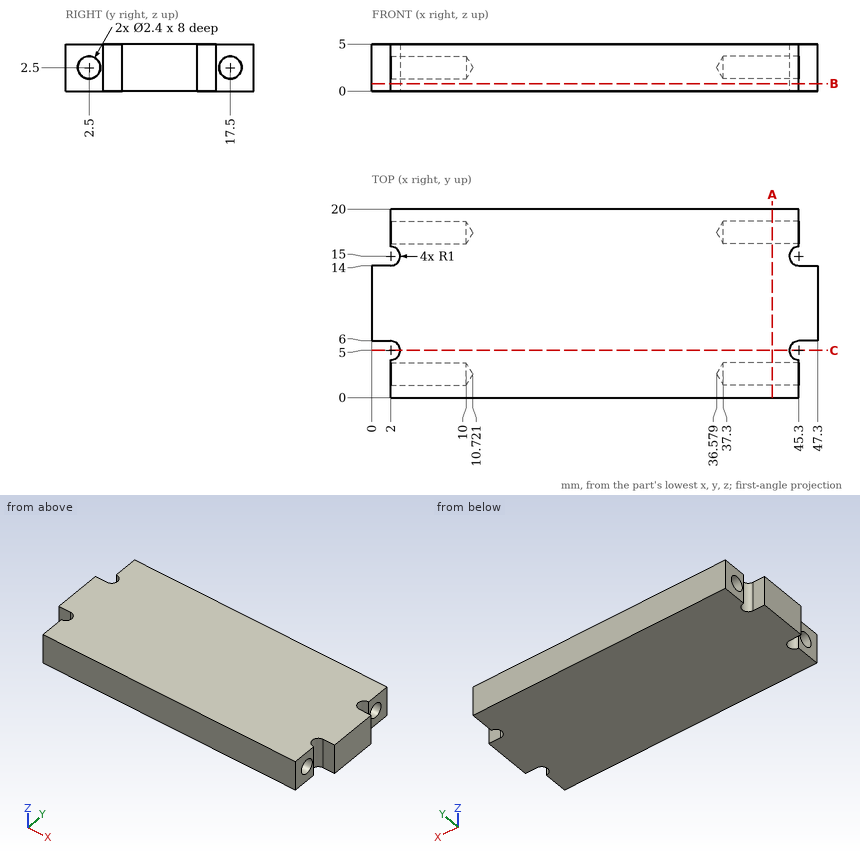
Input: dimensioned drawing with shaded views. Units: mm. Origin: part minimum x, y, z. Give positions to 0.01 mm unless a question says otherwise; leave off trailing zeros. Order: outer loops, then holes, each group sorted by start corner. A loop starts at its lowest first (then second) coordinate and runs counter-clockwise, first axis right, second up. Notation, with made-up numbers: (-23, -28.5) -> (2, -28.5) arc R18 ccw to (2, -12.5) -> close; hole circle Ø2 at (47.5, 58). An arc over 180 degrees is marked (long way). Use one line per item in the form item = value.
1) Section A-A, the plane x = 42.5. Return loops of the section in (y, z).
Response values:
outline = (0, 0) -> (20, 0) -> (20, 5) -> (0, 5) -> close; hole circle Ø2.4 at (2.5, 2.5); hole circle Ø2.4 at (17.5, 2.5)
2) Section B-B, the plane z = 0.8. Return loops of the section in (x, y), and give its area (3 significant figures).
Response values:
outline = (0, 6) -> (2, 6) arc R1 cw to (2, 4) -> (2, 0) -> (45.3, 0) -> (45.3, 4) arc R1 cw to (45.3, 6) -> (47.3, 6) -> (47.3, 14) -> (45.3, 14) arc R1 cw to (45.3, 16) -> (45.3, 20) -> (2, 20) -> (2, 16) arc R1 cw to (2, 14) -> (0, 14) -> close
area = 892 mm^2
3) First-contact query: pin 1 Ø2 at (y, z) = (18, 1.5) entering from +X; pin 2 Ø3 at (y, z) = (17.5, 2.5) entering from -X; pin 3 Ø1.4 at (y, z) = (17.5, 2.5) entering from +X. Flat tips, straight axial feed; report the tip coordinate or a pass-through.
Response values:
pin_1 = 45.3
pin_2 = 2
pin_3 = 37
4) Line query: probe 1 along Y at (x, z) = (41, 2.5); probe 2 along Z at (x, y) = (3.5, 2.5); probe 3 along Y at (x, z) = (7, 2). Output: solid intervals per line, ascending.
Response values:
probe_1 = 0 to 1.3, 3.7 to 16.3, 18.7 to 20
probe_2 = 0 to 1.3, 3.7 to 5
probe_3 = 0 to 1.41, 3.59 to 16.41, 18.59 to 20
5) Section C-C, the plane y = 5. Return loops of the section in (x, z), and give its area (4 significant figures).
Response values:
outline = (3, 0) -> (44.3, 0) -> (44.3, 5) -> (3, 5) -> close
area = 206.5 mm^2
